For this review, take the finished solid that the model builds, in its own axes (mm). A direction names the side the tool comes from. Round coordinates to 2 decimals unless told otherwise and drop trailing zeros. Order: outer loops, then holes, each group sorted by start corner. A loop starts at its lowest first (then second) coordinate and runs counter-clockwise, first axis right, second up. Notation, with made-up numbers: (5.25, 40) -> (50.25, 40) arc R29 cw to (50.25, 65) -> close; hole circle Ø9 at (-6.75, -13). An arc over 180 degrees is marked (long way). Answer in a Markdown table with one row per item.
```python
from build123d import *

# Parameters (mm, degrees)
F0_W        = 52
F0_H        = 12
F1_DEPTH    = 4
F2_R        = 4.1
F2_R_2      = 3.6
F3_DEPTH    = 3
F4_DEPTH    = 25
F5_R        = 5.99999
F6_W        = 30
F6_H        = 4
F7_DEPTH    = 25
F8_T1_DEPTH = 45.3877798739
F9_R        = 5


# Not quite as in the source:
# - a fillet or chamfer that OpenCascade refuses, or shapes differently, is made with other operations: its cross-section is extruded or revolved along the edge and cut away or added
# - a fillet or chamfer is up to 0.001 mm smaller than in the source, because OpenCascade refuses the exact size
# - a feature names something its author has since deleted; it is built from what else it names


with BuildPart() as f1:
    # F0 (on Top) → F1 (new body)
    with BuildSketch(Plane.XY):
        with Locations((6.1197612388, 6)):
            Rectangle(F0_W, F0_H)
    extrude(amount=F1_DEPTH)

    # F2 (on face) → F3 (cut)
    with BuildSketch(Plane.XY.offset(4)):
        with Locations((-13.8802387612, 6)):
            Circle(F2_R)
        with Locations((-13.8802387612, 6)):
            Circle(F2_R_2, mode=Mode.SUBTRACT)
        with Locations((26.1197612388, 6)):
            Circle(F2_R)
        with Locations((26.1197612388, 6)):
            Circle(F2_R_2, mode=Mode.SUBTRACT)
    extrude(amount=-F3_DEPTH, mode=Mode.SUBTRACT)

    # F2 (on face) → F4 (cut)
    with BuildSketch(Plane.XY.offset(4)):
        with Locations((-13.8802387612, 6)):
            Circle(F2_R_2)
        with Locations((26.1197612388, 6)):
            Circle(F2_R_2)
    extrude(amount=-F4_DEPTH, mode=Mode.SUBTRACT)

    # F5 (radius 6 in the source; OpenCascade refuses exactly that, so slightly less here)
    f5_edges = [f1.edges().sort_by_distance(p)[0] for p in [
        (32.119761, 12, 2),
        (32.119761, 0, 2),
        (-19.880239, 12, 2),
        (-19.880239, 0, 2),
    ]]
    fillet(f5_edges, radius=F5_R)

    # F6 (on face) → F7 (cut)
    with BuildSketch(Plane.XY.offset(4)):
        with Locations((6.1197612388, 10)):
            Rectangle(F6_W, F6_H)
        with Locations((6.1197612388, 2)):
            Rectangle(F6_W, F6_H)
    extrude(amount=-F7_DEPTH, mode=Mode.SUBTRACT)

    # F8: fillet of radius 5.5 on 4 edges, made by hand

    # F8_s2 → F8_t1 (cut)
    with BuildSketch(Plane.XY.offset(-20.693889937)):
        with BuildLine():
            ThreePointArc((-17.1042715454, 11.0602033843), (-12.2308229409, 11.5763851223), (-8.8802387612, 8))
            Line((-8.8802387612, 8), (-8.3533713972, 8.1578314949))
            ThreePointArc((-8.3533713972, 8.1578314949), (-8.3302387612, 10), (-8.3302387612, 12))
            Line((-8.3302387612, 12), (-8.8802387612, 12.55))
            ThreePointArc((-8.8802387612, 12.55), (-13.8802487612, 12.55), (-17.3998074599, 11.5240552176))
            Line((-17.3998074599, 11.5240552176), (-17.1042715454, 11.0602033843))
        make_face()
        with BuildLine():
            ThreePointArc((-8.8802387612, 4), (-12.2308229409, 0.4236148777), (-17.1042715454, 0.9397966157))
            Line((-17.1042715454, 0.9397966157), (-17.3998074599, 0.4759447824))
            ThreePointArc((-17.3998074599, 0.4759447824), (-13.8802487612, -0.55), (-8.8802387612, -0.55))
            Line((-8.8802387612, -0.55), (-8.3302387612, 0))
            ThreePointArc((-8.3302387612, 0), (-8.3302387612, 2), (-8.3533713972, 3.8421685051))
            Line((-8.3533713972, 3.8421685051), (-8.8802387612, 4))
        make_face()
        with BuildLine():
            ThreePointArc((29.3437940231, 0.9397966157), (24.4703454185, 0.4236148777), (21.1197612388, 4))
            Line((21.1197612388, 4), (20.5928938749, 3.8421685051))
            ThreePointArc((20.5928938749, 3.8421685051), (20.5697612388, 2), (20.5697612388, 0))
            Line((20.5697612388, 0), (21.1197612388, -0.55))
            ThreePointArc((21.1197612388, -0.55), (26.1197712388, -0.55), (29.6393299376, 0.4759447824))
            Line((29.6393299376, 0.4759447824), (29.3437940231, 0.9397966157))
        make_face()
        with BuildLine():
            ThreePointArc((21.1197612388, 8), (24.4703454185, 11.5763851223), (29.3437940231, 11.0602033843))
            Line((29.3437940231, 11.0602033843), (29.6393299376, 11.5240552176))
            ThreePointArc((29.6393299376, 11.5240552176), (26.1197712388, 12.55), (21.1197612388, 12.55))
            Line((21.1197612388, 12.55), (20.5697612388, 12))
            ThreePointArc((20.5697612388, 12), (20.5697612388, 10), (20.5928938749, 8.1578314949))
            Line((20.5928938749, 8.1578314949), (21.1197612388, 8))
        make_face()
    extrude(amount=F8_T1_DEPTH, mode=Mode.SUBTRACT)

    # F9
    f9_edges = [f1.edges().sort_by_distance(p)[0] for p in [
        (-8.880239, 8, 2),
        (-8.880239, 4, 2),
        (21.119761, 8, 2),
        (21.119761, 4, 2),
    ]]
    fillet(f9_edges, radius=F9_R)


solid = f1.part
```
Q1. The part is to be moulded in two halves that separate along Y. For faces 1 (the face through (31.36, 8.92, 2.03)), 2 (the face through (-17.477, 6.158, 0.507)), 3 (the face through (6, 6, 4)), say which applies: +Y half, -Y half, draft (parallel to the pull), parting line (faces both ways), or undercut.
Answer key:
| item | result |
|---|---|
| face 1 | +Y half |
| face 2 | undercut |
| face 3 | draft |
Q2. To check wall thickness, follow probe 1 along X at (y, z) = (4.75, 3); probe 2 along X at (y, z) = (2.5, 3.8); probe 3 along Y at (x, z) = (10.5, 1.6). State the ranges of each line that lie inside material, in increasing order.
Answer key:
| item | result |
|---|---|
| probe 1 | x = -19.75 to -17.79, -9.98 to 22.21, 30.02 to 31.99 |
| probe 2 | x = -18.75 to -16.02, -11.74 to -9.54, 21.78 to 23.98, 28.26 to 30.99 |
| probe 3 | y = 4 to 8 |
Q3. Clearance check with flat-ended pins moving along their axes: pin 1 Ø1.5 at (y, z) = (3, 3) entering from -X; pin 2 Ø1 at (x, z) = (-4, 1.5) entering from +Y; pin 3 Ø1.2 at (x, z) = (6.5, 2.5) entering from -Y. State where each tip first meets the part, or that it passes through.
Answer key:
| item | result |
|---|---|
| pin 1 | stops at x = -19.44 |
| pin 2 | stops at y = 8 |
| pin 3 | stops at y = 4 |
Q4. Take a section at A-A, the plane x = -11. Write out the cut boundary in (y, z), then the cut area to 3 significant figures.
Answer key:
| item | result |
|---|---|
| outline | (1.07, 0) -> (3.84, 0) -> (3.84, 1) -> (3.08, 1) -> (3.08, 4) -> (1.07, 4) -> close; (8.16, 0) -> (10.93, 0) -> (10.93, 4) -> (8.92, 4) -> (8.92, 1) -> (8.16, 1) -> close |
| area | 17.6 mm^2 |
Q5. Take a section at B-B, the plane z = 0.5. Give the number of separate pieces and of enclosed holes in the cut face, then the cut area to 3 significant figures.
Answer key:
| item | result |
|---|---|
| separate pieces | 1 |
| enclosed holes | 2 |
| area | 252 mm^2 |
Q6. Take a section at C-C, the plane y = 4.75. Write out the cut boundary in (x, z).
Answer key:
| item | result |
|---|---|
| outline | (-19.75, 0) -> (-17.26, 0) -> (-17.26, 1) -> (-17.79, 1) -> (-17.79, 4) -> (-19.75, 4) -> close; (-10.5, 0) -> (22.74, 0) -> (22.74, 1) -> (22.21, 1) -> (22.21, 4) -> (-9.98, 4) -> (-9.98, 1) -> (-10.5, 1) -> close; (29.5, 0) -> (31.99, 0) -> (31.99, 4) -> (30.02, 4) -> (30.02, 1) -> (29.5, 1) -> close |
Q7. Tool access review of faces 4 (the face through (31.36, 3.08, 2.03)), 5 (the face through (-8.1, 3.52, 1.97)), 6 (the face through (-14.769, 1.997, 2.521)), 7 (the face through (-8.154, 8.505, 1.972)): name each direction out of +Z, -Z, +X, -X, +Y, -Y from which nothing blocks a thin tool from reaching the whole face with its end or side.
Answer key:
| item | result |
|---|---|
| face 4 | +Z, -Z, +X, -Y |
| face 5 | +Z, -Z, -Y |
| face 6 | +Z |
| face 7 | +Z, -Z, +Y |
